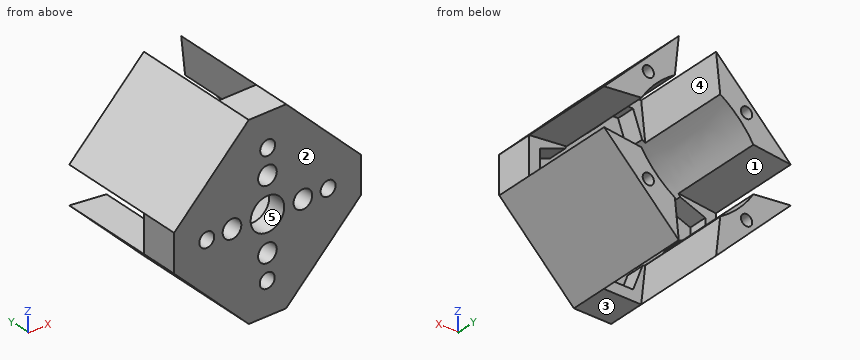
from build123d import *

# Parameters (mm, degrees)
SKETCH1_W           = 50
SKETCH1_H           = 50
SKETCH1_R           = 4.5
BOSS_EXTRUDE1_DEPTH = 5
SKETCH2_R           = 2
CUT_EXTRUDE1_DEPTH  = 36.707142143
BOSS_EXTRUDE2_DEPTH = 30
BOSS_EXTRUDE3_DEPTH = 30
CUT_EXTRUDE5_DEPTH  = 25
SKETCH9_R           = 2.5
CUT_EXTRUDE8_DEPTH  = 47.36809265
SKETCH10_R          = 1.5
CUT_EXTRUDE9_DEPTH  = 10


with BuildPart() as part:
    # Sketch1 → Boss-Extrude1 (new body)
    with BuildSketch(Plane(origin=(0, 0, 0), x_dir=(1, 0, 0), z_dir=(0, 1, 0))):
        Rectangle(SKETCH1_W, SKETCH1_H)
        with Locations(Location((0, 0, 0), (0, 0, 270))):
            Circle(SKETCH1_R, mode=Mode.SUBTRACT)
    extrude(amount=BOSS_EXTRUDE1_DEPTH)

    # Sketch2 → Cut-Extrude1 (cut, through all)
    with BuildSketch(Plane(origin=(0, 5, 0), x_dir=(1, 0, 0), z_dir=(0, 1, 0))):
        with Locations(Location((-0.058911488, 16.249893213, 0), (0, 0, 270))):
            Circle(SKETCH2_R)
        with Locations(Location((16.249893213, -0.058911488, 0), (0, 0, 90))):
            Circle(SKETCH2_R)
        with Locations(Location((0.058911488, -16.249893213, 0), (0, 0, 270))):
            Circle(SKETCH2_R)
        with Locations(Location((-16.249893213, 0.058911488, 0), (0, 0, 90))):
            Circle(SKETCH2_R)
        Polygon((-25, 25), (-25, 5), (-5, 25), align=None)
        Polygon((25, -25), (5, -25), (25, -5), align=None)
        Polygon((-25, -25), (-25, -5), (-5, -25), align=None)
        Polygon((25, 25), (25, 5), (5, 25), align=None)
    extrude(amount=-CUT_EXTRUDE1_DEPTH, mode=Mode.SUBTRACT)

    # Sketch3 → Boss-Extrude2 (add)
    with BuildSketch(Plane(origin=(0, 5, 0), x_dir=(1, 0, 0), z_dir=(0, 1, 0))):
        Polygon((-5, 25), (-7.828427125, 22.171572875), (-22.171572875, 7.828427125), (-25, 5), (-25, -5), (-22.171572875, -7.828427125), (-5, -25), (0, -25), (5, -25), (7.828427125, -22.171572875), (22.171572875, -7.828427125), (25, -5), (25, 5), (7.828427125, 22.171572875), (5, 25), align=None)
        Polygon((-2.828427125, -22.171572875), (-22.171572875, -2.828427125), (-22.171572875, 2.828427125), (-2.828427125, 22.171572875), (2.828427125, 22.171572875), (22.171572875, 2.828427125), (22.171572875, -2.828427125), (2.828427125, -22.171572875), align=None, mode=Mode.SUBTRACT)
    extrude(amount=BOSS_EXTRUDE2_DEPTH)

    # Sketch4 → Boss-Extrude3 (add)
    with BuildSketch(Plane(origin=(0, 35, 0), x_dir=(1, 0, 0), z_dir=(0, 1, 0))):
        with BuildLine():
            add(Edge.make_bspline(
                [(-5.341714296, 15.415645017), (-9.777866181, 12.873181646), (-13.108736095, 9.402087486), (-15.504012831, 5.253346482)],
                knots=[0, 0, 0, 0, 1, 1, 1, 1], degree=3))
            Line((-15.504012831, 5.253346482), (-22.171572875, 2.828427125))
            Line((-22.171572875, 2.828427125), (-2.828427125, 22.171572875))
            Line((-2.828427125, 22.171572875), (-5.341714296, 15.415645017))
        make_face()
        with BuildLine():
            Line((5.341714296, 15.415645017), (2.828427125, 22.171572875))
            Line((2.828427125, 22.171572875), (22.171572875, 2.828427125))
            Line((22.171572875, 2.828427125), (15.504012831, 5.253346482))
            add(Edge.make_bspline(
                [(5.341714296, 15.415645017), (9.777866181, 12.873181646), (13.108736095, 9.402087486), (15.504012831, 5.253346482)],
                knots=[0, 0, 0, 0, 1, 1, 1, 1], degree=3))
        make_face()
        with BuildLine():
            Line((15.415645017, -5.341714296), (22.171572875, -2.828427125))
            Line((22.171572875, -2.828427125), (2.828427125, -22.171572875))
            Line((2.828427125, -22.171572875), (5.253346482, -15.504012831))
            add(Edge.make_bspline(
                [(15.415645017, -5.341714296), (12.873181646, -9.777866181), (9.402087486, -13.108736095), (5.253346482, -15.504012831)],
                knots=[0, 0, 0, 0, 1, 1, 1, 1], degree=3))
        make_face()
        with BuildLine():
            add(Edge.make_bspline(
                [(-15.415645017, -5.341714296), (-12.873181646, -9.777866181), (-9.402087486, -13.108736095), (-5.253346482, -15.504012831)],
                knots=[0, 0, 0, 0, 1, 1, 1, 1], degree=3))
            Line((-5.253346482, -15.504012831), (-2.828427125, -22.171572875))
            Line((-2.828427125, -22.171572875), (-22.171572875, -2.828427125))
            Line((-22.171572875, -2.828427125), (-15.415645017, -5.341714296))
        make_face()
    extrude(amount=-BOSS_EXTRUDE3_DEPTH)

    # Sketch7 → Cut-Extrude5 (cut)
    with BuildSketch(Plane(origin=(0, 35, 0), x_dir=(1, 0, 0), z_dir=(0, 1, 0))):
        Polygon((-25, 5), (-25, -5), (-14.999999986, -6.043670064), (-14.999999986, 6.093977805), align=None)
        Polygon((25, -5), (14.999999986, -6.043670064), (14.999999986, 6.093977805), (25, 5), align=None)
        Polygon((-5, -25), (5, -25), (6.043670064, -14.999999986), (-6.093977805, -14.999999986), align=None)
        Polygon((5, 25), (6.043670064, 14.999999986), (-6.093977805, 14.999999986), (-5, 25), align=None)
    extrude(amount=-CUT_EXTRUDE5_DEPTH, mode=Mode.SUBTRACT)

    # Sketch9 → Cut-Extrude8 (cut, through all)
    with BuildSketch(Plane(origin=(0, 5, 0), x_dir=(1, 0, 0), z_dir=(0, 1, 0))):
        with Locations(Location((0, 9.499893213, 0), (0, 0, 270))):
            Circle(SKETCH9_R)
        with Locations(Location((0, -9.499893213, 0), (0, 0, 90))):
            Circle(SKETCH9_R)
        with Locations(Location((9.499893213, 0, 0), (0, 0, 270))):
            Circle(SKETCH9_R)
        with Locations(Location((-9.499893213, 0, 0), (0, 0, 90))):
            Circle(SKETCH9_R)
    extrude(amount=-CUT_EXTRUDE8_DEPTH, mode=Mode.SUBTRACT)

    # Sketch10 → Cut-Extrude9 (cut)
    with BuildSketch(Plane(origin=(0, 35, 0), x_dir=(1, 0, 0), z_dir=(0, 1, 0))):
        with Locations(Location((13.166804189, 13.166804189, 0), (0, 0, 270))):
            Circle(SKETCH10_R)
        with Locations(Location((-13.166804189, 13.166804189, 0), (0, 0, 90))):
            Circle(SKETCH10_R)
        with Locations(Location((-13.166804189, -13.166804189, 0), (0, 0, 270))):
            Circle(SKETCH10_R)
        with Locations(Location((13.166804189, -13.166804189, 0), (0, 0, 90))):
            Circle(SKETCH10_R)
    extrude(amount=-CUT_EXTRUDE9_DEPTH, mode=Mode.SUBTRACT)


solid = part.part
Part model, mm, in its own coordinate system. Face numbers are marked on the shaded views. A direction names the side the tool comes from. Coordinates: 2 decimals unless noted, no trailing zeros. Write each loop counter-clockwise with the first axis right and the second up, starting at its lowest first coordinate (ties: lowest second). Pieces come first, ordered by that corner, then holes. Notation, with made-up numbers: (71, 68) - (81, 68) arc R17 ccw to (81, 90) - close; hole circle Ø1 at (-31, 68). An arc over 180 degrees is marked (long way). Put each result on its own line as item: value.
1. Probe line 1 along X through (y, z) = (2, 0.5); line 2 along Y through (x, z) = (-10, -2.5); line 3 along Z through (x, y) = (-11, 31). List the from-to ranges inside material, lowest first. Write a range as [from, to].
Final values:
line 1: x = [-25, -18.17], [-14.33, -11.95], [-7.05, -4.47], [4.47, 7.05], [11.95, 14.3], [18.2, 25]
line 2: y = [0, 5]
line 3: z = [-19, -11.13], [11.13, 19]
2. Flat gauge pins, fed straight in: pin 1 Ø10 at (y, z) = (26.5, 18) entering from -X; pin 2 Ø3 at (x, z) = (20, -1.5) entering from +Y; pin 3 Ø10 at (y, z) = (17.5, -11.5) entering from +X. Where does each tip first touch, or does it go through?
Final values:
pin 1: stops at x = -17
pin 2: stops at y = 5
pin 3: stops at x = 23.5
3. Band-saw the part on C-C (y = 3.5). Give the number of separate pieces and of enclosed holes in the cut face, then the cut area to 3 significant figures.
Final values:
separate pieces: 1
enclosed holes: 9
area: 1,510 mm²
4. Two-plate mould, pull along Z, no slides. Class the marked faces 1, 2 and 3: +Z half, -Z half, draft (parallel to the pull), parting line (faces both ways), or undercut.
Final values:
face 1: undercut
face 2: draft
face 3: -Z half
5. Band-saw the part on A-A (x = 1). Write the cut outline in (y, z).
Final values:
outline: (0, -25) - (10, -25) - (10, -22.17) - (5, -22.17) - (5, -17.95) - (0, -17.95) - close; (0, -14.55) - (5, -14.55) - (5, -11.79) - (0, -11.79) - close; (0, -7.21) - (5, -7.21) - (5, -4.39) - (0, -4.39) - close; (0, 4.39) - (5, 4.39) - (5, 7.21) - (0, 7.21) - close; (0, 11.79) - (5, 11.79) - (5, 14.49) - (0, 14.49) - close; (0, 18.01) - (5, 18.01) - (5, 22.17) - (10, 22.17) - (10, 25) - (0, 25) - close
6. 3-axis set-ups, long thin cutter, end or side, ignore diameter. For the marked faces 4 and 5: which of +Z, -Z, +X, -X, +Y, -Y reach the whole face in a straight line?
Final values:
face 4: +Y
face 5: +Y, -Y
7. Band-saw the part on B-B (z = 0.5). Write the cut outline in (x, y), then the cut area to 3 significant figures.
Final values:
outline: (-25, 0) - (-18.17, 0) - (-18.17, 5) - (-22.17, 5) - (-22.17, 10) - (-25, 10) - close; (-14.33, 0) - (-11.95, 0) - (-11.95, 5) - (-14.33, 5) - close; (-7.05, 0) - (-4.47, 0) - (-4.47, 5) - (-7.05, 5) - close; (4.47, 0) - (7.05, 0) - (7.05, 5) - (4.47, 5) - close; (11.95, 0) - (14.3, 0) - (14.3, 5) - (11.95, 5) - close; (18.2, 0) - (25, 0) - (25, 10) - (22.17, 10) - (22.17, 5) - (18.2, 5) - close
area: 146 mm²
